Here's how the part is built. I have some questions about the finished solid (model axes, mm). A direction names the side the tool comes from. Coordinates: 2 decimals unless noted, no trailing zeros. Loops run counter-clockwise (first coordinate to the right, second up) from the corner with the lowest first, then second, coordinate; pieces in that order, holes last.
from build123d import *

# Parameters (mm, degrees)
SKETCH_W        = 9.98
SKETCH_H        = 9.98
PAD_DEPTH       = 45
SKETCH001_W     = 7
SKETCH001_H     = 7
POCKET_DEPTH    = 8.5
PAD001_DEPTH    = 12
FILLET_R        = 1
SKETCH004_W     = 35
SKETCH004_H     = 9.98
POCKET002_DEPTH = 6
CHAMFER_SIZE    = 1.4
PAD002_DEPTH    = 4
FILLET001_R     = 1.5


with BuildPart() as part:
    # Sketch → Pad (new body)
    with BuildSketch(Plane.XZ):
        Rectangle(SKETCH_W, SKETCH_H)
    extrude(amount=PAD_DEPTH)

    # Sketch001 (on Face3 of Pad) → Pocket (cut)
    with BuildSketch(Plane.YZ.offset(4.99)):
        with Locations((-36.5, -1.49)):
            Rectangle(SKETCH001_W, SKETCH001_H)
    extrude(amount=-POCKET_DEPTH, mode=Mode.SUBTRACT)

    # Sketch002 (on Face4 of Pocket) → Pad001 (join)
    with BuildSketch(Plane(origin=(0, 0, 0), x_dir=(-1, 0, 0), z_dir=(0, 1, 0))):
        Polygon((-4.99, 2.5), (-2.5, 4.99), (2.5, 4.99), (4.99, 2.5), (4.99, -2.5), (2.5, -4.99), (-2.5, -4.99), (-4.99, -2.5), align=None)
    extrude(amount=PAD001_DEPTH)

    # Fillet
    fillet_edges = [part.edges().sort_by_distance(p)[0] for p in [
        (3.745, 12, 3.745),
        (0, 12, 4.99),
        (-3.745, 12, 3.745),
        (-4.99, 12, 0),
        (-3.745, 12, -3.745),
        (0, 12, -4.99),
        (3.745, 12, -3.745),
        (4.99, 12, 0),
    ]]
    fillet(fillet_edges, radius=FILLET_R)

    # Sketch004 → Pocket002 (cut)
    with BuildSketch(Plane.YZ.offset(4.99)):
        with Locations((-27.5, 0)):
            Rectangle(SKETCH004_W, SKETCH004_H)
    extrude(amount=-POCKET002_DEPTH, mode=Mode.SUBTRACT)

    # Chamfer
    chamfer_edges = [part.edges().sort_by_distance(p)[0] for p in [
        (4.99, -10, 0),
    ]]
    chamfer(chamfer_edges, length=CHAMFER_SIZE)

    # Sketch005 → Pad002 (join)
    with BuildSketch(Plane.XZ):
        Polygon((4.99, 1.5), (6.99, 1.5), (6.99, -1.5), (4.99, -1.5), (4.99, 0), align=None)
    extrude(amount=-PAD002_DEPTH)

    # Fillet001
    fillet001_edges = [part.edges().sort_by_distance(p)[0] for p in [
        (6.99, 4, 0),
    ]]
    fillet(fillet001_edges, radius=FILLET001_R)


solid = part.part
Q1. Please list where these lines run through material, in increasing order: probe 1 along Y at (x, z) = (-2, 0.75); probe 2 along X at (y, z) = (-33.5, -3.5); probe 3 along X at (y, z) = (-25, 4.5).
Q2. For faces 4 (the flat face through (-1.01, -28, 0)), 5 (the flat face through (3.73, 5.42, -3.76)), 6 (the flat face through (-2, -33, -2)), which set-ups out of +Z, -Z, +X, -X, +Y, -Y let a thin tool reach every point of the face, with its end or its side?
Q3. Suppose I cut it at C-C on z = 0. Write out the boundary of the cut face in (x, y).
Q4. Suppose I cut it at A-A on x = -1.5. Write out the boundary of the cut face in (y, z).
Q5. We'd pull the mould along Y, two halves only. Please class faces 1 (the flat face through (-2, -37, 2.01)), 2 (the flat face through (1, -10, 0)), 3 (the flat face through (0, 12, 0)): pulls with the +Y half, pulls with the -Y half, needs draft (parallel to the pull), parting line crosses it, or undercut.
Q6. Will these pins go through, and if not, where does the flat tip stop? P1, Ø1.4, axis at x = 0.5, z = -1, coming from the -Y side; P2, Ø1, axis at y = -33, z = 3, coming from the +X side; P3, Ø4, axis at x = 5.5, y = -12, coming from the -Z side; P4, Ø0.7, axis at x = -3, z = 4.5, coming from the +Y side.
Q7. Suppose I cut it at D-D on y = -35. Write out the boundary of the cut face in (x, z), and give its area (3 significant figures).
Q8. Suppose I cut it at B-B on y = 4.5. Write out the boundary of the cut face in (x, z).
Check values:
1. probe 1: y = -45 to -40, -33 to 12
1. probe 2: x = -4.99 to -3.51
1. probe 3: x = -4.99 to -1.01
2. face 4: +Z, -Z, +X, -Y
2. face 5: -Z, +X, +Y
2. face 6: -Z, +X
3. outline: (-4.99, -45) - (-1.01, -45) - (-1.01, -40) - (-3.51, -40) - (-3.51, -33) - (-1.01, -33) - (-1.01, -10) - (3.59, -10) - (4.99, -8.6) - (4.99, 0) - (6.99, 0) - (6.99, 2.5) arc R1.5 ccw to (5.49, 4) - (4.99, 4) - (4.99, 11) arc R1 ccw to (3.99, 12) - (-3.99, 12) arc R1 ccw to (-4.99, 11) - close
4. outline: (-45, -4.99) - (-40, -4.99) - (-40, 2.01) - (-33, 2.01) - (-33, -4.99) - (11, -4.99) arc R1 ccw to (12, -3.99) - (12, 3.99) arc R1 ccw to (11, 4.99) - (-45, 4.99) - close
5. face 1: undercut
5. face 2: pulls with the -Y half
5. face 3: pulls with the +Y half
6. P1: stops at y = -10
6. P2: stops at x = -1.01
6. P3: passes through
6. P4: stops at y = 11.75
7. outline: (-4.99, -4.99) - (-3.51, -4.99) - (-3.51, 2.01) - (-1.01, 2.01) - (-1.01, 4.99) - (-4.99, 4.99) - close
7. area: 22.2 mm2
8. outline: (-4.99, -2.5) - (-2.5, -4.99) - (2.5, -4.99) - (4.99, -2.5) - (4.99, 2.5) - (2.5, 4.99) - (-2.5, 4.99) - (-4.99, 2.5) - close
